from build123d import *

# Parameters (mm, degrees)
F1_DEPTH = 1407
F2_R     = 85
F3_R     = 50


with BuildPart() as f1:
    # F0 (on Front) → F1 (new body)
    with BuildSketch(Plane.XZ):
        Polygon((0, 615), (0, 0), (1020, 0), (1020, 250), (485, 250), (275, 615), align=None)
    extrude(amount=F1_DEPTH)

    # F2
    f2_edges = [f1.edges().sort_by_distance(p)[0] for p in [
        (275, -703.5, 615),
        (1020, -703.5, 250),
        (1020, -703.5, 0),
        (0, -703.5, 0),
        (0, -703.5, 615),
    ]]
    fillet(f2_edges, radius=F2_R)

    # F3
    f3_edges = [f1.edges().sort_by_distance(p)[0] for p in [
        (392.257957, 0, 411.194503),
        (155.419892, 0, 615),
        (268.395245, 0, 603.580111),
        (710, 0, 250),
        (995.104076, 0, 225.104076),
        (1020, 0, 125),
        (995.104076, 0, 24.895924),
        (24.895924, 0, 590.104076),
        (0, 0, 307.5),
        (24.895924, 0, 24.895924),
        (510, 0, 0),
        (710, -1407, 250),
        (392.257957, -1407, 411.194503),
        (268.395245, -1407, 603.580111),
        (155.419892, -1407, 615),
        (24.895924, -1407, 590.104076),
        (0, -1407, 307.5),
        (24.895924, -1407, 24.895924),
        (510, -1407, 0),
        (995.104076, -1407, 24.895924),
        (1020, -1407, 125),
        (995.104076, -1407, 225.104076),
    ]]
    fillet(f3_edges, radius=F3_R)


solid = f1.part
Geometry: final body of the model. Coordinates: model frame, mm. A direction names the side the tool comes from. Give positions to 0.01 mm unless a question says otherwise; leave off trailing zeros. Write each loop counter-clockwise with the first axis right and the second up, starting at its lowest first coordinate (ties: lowest second). Pieces come first, ordered by that corner, then holes. Notation, with made-up numbers: M 30,85.25 L 84,85.25 A35 cw 84,118.25 Z; hole C -3,25 d9. An arc over 180 degrees is marked long. Answer in a Markdown table with one row per item. Add a question column.
(1) Ray query, line 1 (Z direction, x = 492.5, y = -1134.5); line 2 (X direction, y = -486, z = 171); line 3 (X direction, y = -629, z = 71). Return the intervals inside material, ascending.
(2) Section A-A on y = -513. Return loops of the section in (x, z).
(3) First-contact query: pin 1 (8 mm diameter, centred on y = -435, z = 544, fed in from -X); pin 2 (1.5 mm diameter, centred on x = 591, y = -694, fed in from +Z). Flat tips, straight axial feed; report the tip coordinate or a pass-through.
(4) Reachability of faces 1 (the cylindrical face through (692.189, -1392.742, 234.964)), 2 (the cylindrical face through (692.189, -14.258, 234.964)), 3 (the flat face through (713, -694, 250)) from +Z, -Z, +X, -X, +Y, -Y: full face, straight path, thin tool, end or side. Return the list, or none.
(5) Section B-B on x = 727. Return loops of the section in (y, z), and give its area (3 significant figures).
Result set:
| question | item | result |
|---|---|---|
| 1 | line 1 | z = 0 to 250 |
| 1 | line 2 | x = 0 to 1019.79 |
| 1 | line 3 | x = 1.16 to 1018.84 |
| 2 | outline | M 0,85 A85 ccw 85,0 L 935,0 A85 ccw 1020,85 L 1020,165 A85 ccw 935,250 L 485,250 L 299.52,572.39 A85 ccw 225.84,615 L 85,615 A85 ccw 0,530 Z |
| 3 | pin 1 | stops at x = 0.59 |
| 3 | pin 2 | stops at z = 250 |
| 4 | face 1 | +Z, +X, -Y |
| 4 | face 2 | +Z, +X, +Y |
| 4 | face 3 | +Z, +X, +Y, -Y |
| 5 | outline | M -1407,50 A50 ccw -1357,0 L -50,0 A50 ccw 0,50 L 0,200 A50 ccw -50,250 L -1357,250 A50 ccw -1407,200 Z |
| 5 | area | 350,000 mm^2 |
